```python
from build123d import *

# Parameters (mm, degrees)
SKETCH_1_W          = 77
SKETCH_1_H          = 81
EXTRUDE_1_DEPTH     = 20
FILLET_1_R          = 10
FILLET_2_R          = 3
SKETCH_3_R          = 35.5
EXTRUDE_2_DEPTH     = 20
FILLET_3_R          = 1
SKETCH_4_R          = 1.5
CUT_EXTRUDE_1_DEPTH = 10
CUT_EXTRUDE_2_DEPTH = 1
CUT_EXTRUDE_3_DEPTH = 1


with BuildPart() as part:
    # 草图1 → 凸台-拉伸1 (new body)
    with BuildSketch(Plane.XY):
        Rectangle(SKETCH_1_W, SKETCH_1_H)
    extrude(amount=EXTRUDE_1_DEPTH)

    # 圆角1
    fillet_1_edges = [part.edges().sort_by_distance(p)[0] for p in [
        (38.5, -40.5, 10),
        (-38.5, -40.5, 10),
        (-38.5, 40.5, 10),
        (38.5, 40.5, 10),
    ]]
    fillet(fillet_1_edges, radius=FILLET_1_R)

    # 圆角2
    fillet_2_edges = [part.edges().sort_by_distance(p)[0] for p in [
        (38.5, 0, 20),
        (0, -40.5, 20),
        (0, 40.5, 20),
        (-38.5, 0, 20),
        (-35.571067812, 37.571067812, 20),
        (-35.571067812, -37.571067812, 20),
        (35.571067812, 37.571067812, 20),
        (35.571067812, -37.571067812, 20),
    ]]
    fillet(fillet_2_edges, radius=FILLET_2_R)

    # 草图3 → 凸台-拉伸2 (add)
    with BuildSketch(Plane.XY.offset(20)):
        Circle(SKETCH_3_R)
    extrude(amount=EXTRUDE_2_DEPTH)

    # 圆角3
    fillet_3_edges = [part.edges().sort_by_distance(p)[0] for p in [
        (4e-08, 35.5, 20),
        (-4e-08, -35.5, 20),
        (-35.5, 0, 40),
    ]]
    fillet(fillet_3_edges, radius=FILLET_3_R)

    # 草图4 → 切除-拉伸1 (cut)
    with BuildSketch(Plane.XY.offset(40)):
        Circle(SKETCH_4_R)
    extrude(amount=-CUT_EXTRUDE_1_DEPTH, mode=Mode.SUBTRACT)

    # 草图5 → 切除-拉伸2 (cut)
    with BuildSketch(Plane(origin=(0, 40.5, 0), x_dir=(1, 0, 0), z_dir=(0, 1, 0))):
        with BuildLine():
            Line((-10, -6), (10, -6))
            ThreePointArc((10, -6), (14, -10), (10, -14))
            Line((10, -14), (-10, -14))
            ThreePointArc((-10, -14), (-14, -10), (-10, -6))
        make_face()
    extrude(amount=-CUT_EXTRUDE_2_DEPTH, mode=Mode.SUBTRACT)

    # 草图6 → 切除-拉伸3 (cut)
    with BuildSketch(Plane.XY.offset(40)):
        Polygon((0, 27.472496233), (-1.5, 24.874420022), (1.5, 24.874420022), align=None)
    extrude(amount=-CUT_EXTRUDE_3_DEPTH, mode=Mode.SUBTRACT)


solid = part.part
```
Here's how the part is built. I have some questions about the finished solid (model axes, mm). A direction names the side the tool comes from. Give positions to 0.01 mm unless a question says otherwise; leave off trailing zeros. Write each loop counter-clockwise with the first axis right and the second up, starting at its lowest first coordinate (ties: lowest second). Pieces come first, ordered by that corner, then holes.
(1) Imagine slicing it at B-B, the plane z = 36. Write out the boundary of the cut face in (x, y), and give its area (3 significant figures).
Output values:
outline: circle Ø71 at (0, 0); hole circle Ø3 at (0, 0)
area: 3,950 mm2
(2) Thinking about a two-plate mould opening in Y: for faces 6 (the face through (0, 40.5, 5)), 7 (the face through (-1.5, 0.07, 35.07)), 8 (the face through (14, 40, 10)), 9 (the face through (0, 26, 39)), which applies, pulls with the +Y half, pulls with the -Y half, needs draft (parallel to the pull), parting line crosses it, or undercut?
Output values:
face 6: pulls with the +Y half
face 7: undercut
face 8: needs draft
face 9: undercut
(3) If I drill on L1, parallel to Y at x = 0, z = 32.75; L2, parallel to Y at x = 2, z = 11.5; L3, parallel to Z at x = 34.5, y = -28.5, over which ranges is the centre line in solid material (lowest first)?
Output values:
L1: y = -35.5 to -1.5, 1.5 to 35.5
L2: y = -40.5 to 39.5
L3: z = 0 to 20
(4) Will these pins go through, and if not, where does the flat tip stop? pin 1 (0.8 mm diameter, centred on x = 4.5, y = 40, fed in from +Z); pin 2 (4 mm diameter, centred on x = 0, y = 0, fed in from +Z); pin 3 (1.5 mm diameter, centred on x = 26.5, z = 29.5, fed in from -Y); pin 4 (10 mm diameter, centred on y = 9, z = 33, fed in from +X).
Output values:
pin 1: stops at z = 19.14
pin 2: stops at z = 40
pin 3: stops at y = -24.44
pin 4: stops at x = 35.27
(5) Imagine slicing it at A-A, the plane z = 11. Write out the boundary of the cut face in (x, y).
Output values:
outline: (-38.5, -30.5) arc R10 ccw to (-28.5, -40.5) - (28.5, -40.5) arc R10 ccw to (38.5, -30.5) - (38.5, 30.5) arc R10 ccw to (28.5, 40.5) - (13.87, 40.5) - (13.87, 39.5) - (-13.87, 39.5) - (-13.87, 40.5) - (-28.5, 40.5) arc R10 ccw to (-38.5, 30.5) - close
(6) On a 3-axis mill with a long thin cutter (end or side, diameter ignored), from which of +Z, -Z, +X, -X, +Y, -Y can I reach the whole of each face in a straight line? I mean faces 1 (the face through (-14, 40, 10)), 2 (the face through (0.4, -39.6, 19.14)), 3 (the face through (0, 37, 20)), 4 (the face through (2, -37, 20)), 5 (the face through (-0.4, 39.6, 19.14)). Say none if no direction works.
Output values:
face 1: +Y
face 2: +Z, +X, -X, -Y
face 3: +Z, +Y
face 4: +Z, -Y
face 5: +Z, +X, -X, +Y
(7) Imagine slicing it at C-C, the plane z = 18.5. Write out the boundary of the cut face in (x, y), and give its area (3 significant figures).
Output values:
outline: (-38.1, -30.5) arc R9.6 ccw to (-28.5, -40.1) - (28.5, -40.1) arc R9.6 ccw to (38.1, -30.5) - (38.1, 30.5) arc R9.6 ccw to (28.5, 40.1) - (-28.5, 40.1) arc R9.6 ccw to (-38.1, 30.5) - close
area: 6,030 mm2
